from build123d import *

# Parameters (mm, degrees)
SKETCH1_W            = 27.6032
SKETCH1_H            = 35.3248
SKETCH1_W_2          = 25.6032
SKETCH1_H_2          = 33.3248
MAINCASING_DEPTH     = 12.93
SKETCH2_W            = 6.35
SKETCH2_H            = 9.525
SKETCH2_R            = 1.4732
MOUNTINGTABS_DEPTH   = 1.5875
SKETCH3_W            = 3.683
SKETCH3_H            = 7.112
SKETCH3_W_2          = 4.572
SKETCH3_H_2          = 4.572
SKETCH3_R            = 1.1303
BOSS_EXTRUDE3_DEPTH  = 12.93
SKETCH4_W            = 27.6032
SKETCH4_H            = 35.3248
SKETCH4_W_2          = 25.6032
SKETCH4_H_2          = 33.3248
BOSS_EXTRUDE4_DEPTH  = 1.6002
SKETCH5_R            = 1.1303
UPPERHOLES_DEPTH     = 38.848662667
SKETCH6_W            = 25.6032
SKETCH6_H            = 1
BOSS_EXTRUDE5_DEPTH  = 12.93
SKETCH7_W            = 27.6032
SKETCH7_H            = 1
CUT_EXTRUDE2_DEPTH   = 38.848662667
SKETCH8_W            = 47.196128447
SKETCH8_H            = 36.476203794
TEMPMATREMOVAL_DEPTH = 7.62


with BuildPart() as part:
    # Sketch1 → mainCasing (new body)
    with BuildSketch(Plane(origin=(0, 0, 0), x_dir=(1, 0, 0), z_dir=(0, 1, 0))):
        with Locations((2.873828571, -8.628742857)):
            Rectangle(SKETCH1_W, SKETCH1_H)
        with Locations((2.873828571, -8.628742857)):
            Rectangle(SKETCH1_W_2, SKETCH1_H_2, mode=Mode.SUBTRACT)
    extrude(amount=-MAINCASING_DEPTH)

    # Sketch2 → mountingTabs (add)
    # profile 1 of 2: a face of its own
    with BuildSketch(Plane.XZ.offset(12.93)):
        with Locations((-14.102771429, 8.628742857)):
            Rectangle(SKETCH2_W, SKETCH2_H)
        with Locations(Location((-14.102771429, 8.628742857, 0), (0, 0, 270))):
            Circle(SKETCH2_R, mode=Mode.SUBTRACT)
    # profile 2 of 2: a face of its own
    with BuildSketch(Plane.XZ.offset(12.93)):
        with Locations((19.850428571, 8.628742857)):
            Rectangle(SKETCH2_W, SKETCH2_H)
        with Locations(Location((19.850428571, 8.628742857, 0), (0, 0, 270))):
            Circle(SKETCH2_R, mode=Mode.SUBTRACT)
    extrude(amount=-MOUNTINGTABS_DEPTH)

    # Sketch3 → Boss-Extrude3 (add)
    # profile 1 of 4: a face of its own
    with BuildSketch(Plane(origin=(0, 0, 0), x_dir=(1, 0, 0), z_dir=(0, 1, 0))):
        with Locations((-8.086271429, 4.477657143)):
            Rectangle(SKETCH3_W, SKETCH3_H)
    # profile 2 of 4: a face of its own
    with BuildSketch(Plane(origin=(0, 0, 0), x_dir=(1, 0, 0), z_dir=(0, 1, 0))):
        with Locations((13.833928571, 4.477657143)):
            Rectangle(SKETCH3_W, SKETCH3_H)
    # profile 3 of 4: a face of its own
    with BuildSketch(Plane(origin=(0, 0, 0), x_dir=(1, 0, 0), z_dir=(0, 1, 0))):
        with Locations((-7.641771429, -19.703142857)):
            Rectangle(SKETCH3_W_2, SKETCH3_H_2)
        with Locations(Location((-7.235371429, -19.703142857, 0), (0, 0, 270))):
            Circle(SKETCH3_R, mode=Mode.SUBTRACT)
    # profile 4 of 4: a face of its own
    with BuildSketch(Plane(origin=(0, 0, 0), x_dir=(1, 0, 0), z_dir=(0, 1, 0))):
        with Locations((13.389428571, -19.703142857)):
            Rectangle(SKETCH3_W_2, SKETCH3_H_2)
        with Locations(Location((12.983028571, -19.703142857, 0), (0, 0, 270))):
            Circle(SKETCH3_R, mode=Mode.SUBTRACT)
    extrude(amount=-BOSS_EXTRUDE3_DEPTH)

    # Sketch4 → Boss-Extrude4 (add)
    with BuildSketch(Plane(origin=(0, 0, 0), x_dir=(1, 0, 0), z_dir=(0, 1, 0))):
        with Locations((2.873828571, -8.628742857)):
            Rectangle(SKETCH4_W, SKETCH4_H)
        with Locations((2.873828571, -8.628742857)):
            Rectangle(SKETCH4_W_2, SKETCH4_H_2, mode=Mode.SUBTRACT)
    extrude(amount=BOSS_EXTRUDE4_DEPTH)

    # Sketch5 → upperHoles (cut, through all)
    with BuildSketch(Plane.XZ.offset(12.93)):
        with Locations((-7.235371429, -5.239657143)):
            Circle(SKETCH5_R)
        with Locations((12.983028571, -4.731657143)):
            Circle(SKETCH5_R)
    extrude(amount=-UPPERHOLES_DEPTH, mode=Mode.SUBTRACT)

    # Sketch6 → Boss-Extrude5 (add)
    with BuildSketch(Plane.XZ.offset(12.93)):
        with Locations((2.873828571, 12.786342857)):
            Rectangle(SKETCH6_W, SKETCH6_H)
    extrude(amount=-BOSS_EXTRUDE5_DEPTH)

    # Sketch7 → Cut-Extrude2 (cut, through all)
    with BuildSketch(Plane.XZ.offset(12.93)):
        with Locations((2.873828571, 25.791142857)):
            Rectangle(SKETCH7_W, SKETCH7_H)
    extrude(amount=-CUT_EXTRUDE2_DEPTH, mode=Mode.SUBTRACT)

    # Sketch8 → tempMatRemoval (cut)
    with BuildSketch(Plane.XZ.offset(12.93)):
        with Locations((2.61294545, 8.081309562)):
            Rectangle(SKETCH8_W, SKETCH8_H)
    extrude(amount=-TEMPMATREMOVAL_DEPTH, mode=Mode.SUBTRACT)


solid = part.part
Part model, mm, in its own coordinate system. A direction names the side the tool comes from. Give positions to 0.01 mm unless a question says otherwise; leave off trailing zeros. Loops run counter-clockwise (first coordinate to the right, second up) from the corner with the lowest first, then second, coordinate; pieces in that order, holes last.
(1) 3-axis set-ups, long thin cutter, end or side, ignore diameter. For faces 5 (the flat face through (13, -3, 21.989)), 6 (the flat face through (2.8, 1.6, -8.5)), 7 (the flat face through (3, 0, 13)), 8 (the flat face through (-8, -3, -0.922)), 9 (the flat face through (-9.928, -1, 9)): which of +Z, -Z, +X, -X, +Y, -Y reach the whole face in a straight line?
Return value:
face 5: +Z, +Y, -Y
face 6: +Z, -Z, +X, -X, +Y
face 7: +Z, +Y
face 8: +Y, -Y
face 9: +Y
(2) Band-saw the part on B-B (x = -4.5). Write the cut outline in (y, z), and give its area (3 significant figures).
Return value:
outline: (-5.31, -9.03) - (1.6, -9.03) - (1.6, -8.03) - (-5.31, -8.03) - close; (-5.31, 12.29) - (0, 12.29) - (0, 13.29) - (-5.31, 13.29) - close
area: 12.2 mm2
(3) Pin check, flat tips, straight feed: pin 1 (3 mm diameter, centred on x = 12.98, z = -4.73, fed in from +Y); pin 2 (1.1 mm diameter, centred on x = -8.5, y = -2, fed in from +Z); pin 3 (2.5 mm diameter, centred on x = 7, y = -2.5, fed in from +Z). Stop position of each tip, or through.
Return value:
pin 1: stops at y = 0
pin 2: stops at z = 21.99
pin 3: stops at z = 13.29
(4) Band-saw the part on C-C (z = -1.5). Write the cut outline in (x, y), and give its area (3 significant figures).
Return value:
outline: (-10.93, -5.31) - (-6.24, -5.31) - (-6.24, 0) - (-9.93, 0) - (-9.93, 1.6) - (-10.93, 1.6) - close; (11.99, -5.31) - (16.68, -5.31) - (16.68, 1.6) - (15.68, 1.6) - (15.68, 0) - (11.99, 0) - close
area: 52.9 mm2
(5) Pull direction Z, two halves, no side cores. Call faces 1 (the flat face through (15, 0, -5)), 2 (the flat face through (3, -2, -9.034)), 3 (the flat face through (-6.245, -3, -3)), 4 (the flat face through (16, -2, 25.291)): pulls with the +Z half, pulls with the -Z half, needs draft (parallel to the pull), parting line crosses it, or undercut.
Return value:
face 1: needs draft
face 2: pulls with the -Z half
face 3: undercut
face 4: pulls with the +Z half
(6) Band-saw the part on D-D (y = 0.75). Write the cut outline in (x, z), and give its area (3 significant figures).
Return value:
outline: (-10.93, -9.03) - (16.68, -9.03) - (16.68, 25.29) - (15.68, 25.29) - (15.68, -8.03) - (-9.93, -8.03) - (-9.93, 25.29) - (-10.93, 25.29) - close
area: 94.3 mm2
(7) Band-saw the part on A-A (x = -9). Write the cut outline in (y, z), and give its area (3 significant figures).
Return value:
outline: (-5.31, -9.03) - (1.6, -9.03) - (1.6, -8.03) - (0, -8.03) - (0, -0.92) - (-5.31, -0.92) - close; (-5.31, 12.29) - (0, 12.29) - (0, 13.29) - (-5.31, 13.29) - close; (-5.31, 17.42) - (0, 17.42) - (0, 21.99) - (-5.31, 21.99) - close
area: 74.3 mm2
(8) Drill centre lines: line 1 along X through (y, z) = (-2, 0); line 2 along Z through (x, y) = (-0.75, -1.5); line 3 along Z through (x, y) = (15.25, -4.5). Where is each one in solid material? Low to high.
Return value:
line 1: x = -10.93 to -9.93, 15.68 to 16.68
line 2: z = -9.03 to -8.03, 12.29 to 13.29
line 3: z = -9.03 to -0.92, 12.29 to 13.29, 17.42 to 21.99
